```python
from build123d import *

# Parameters (mm, degrees)
SKETCH1_W           = 193
SKETCH1_H           = 10
BOSS_EXTRUDE1_DEPTH = 6
SKETCH4_W           = 16.888888889
SKETCH4_H           = 6
BOSS_EXTRUDE3_DEPTH = 6


with BuildPart() as part:
    # Sketch1 → Boss-Extrude1 (new body)
    with BuildSketch(Plane(origin=(0, 0, 0), x_dir=(1, 0, 0), z_dir=(0, 1, 0))):
        Rectangle(SKETCH1_W, SKETCH1_H)
    extrude(amount=BOSS_EXTRUDE1_DEPTH)

    # Sketch4 → Boss-Extrude3 (add)
    with BuildSketch(Plane.XZ):
        with Locations((-16.888888889, 8)):
            Rectangle(SKETCH4_W, SKETCH4_H)
        with Locations((-50.666666667, 8)):
            Rectangle(SKETCH4_W, SKETCH4_H)
    boss_extrude3 = extrude(amount=-BOSS_EXTRUDE3_DEPTH)

    # Mirror1: Boss-Extrude3 across plane
    add(boss_extrude3.mirror(Plane(origin=(0, 0, 0), x_dir=(0, 0, 1), z_dir=(1, 0, 0))))


solid = part.part
```
Input: part model. Units: mm. Frame: model coordinates. A direction names the side the tool comes from. Give positions to 0.01 mm unless a question says otherwise; leave off trailing zeros. Loops run counter-clockwise (first coordinate to the right, second up) from the corner with the lowest first, then second, coordinate; pieces in that order, holes last.
1) Section query B-B on y = 1.95. Return the cut outline in (x, z), and give its area (3 significant figures).
A:
outline: (-96.5, -5) - (96.5, -5) - (96.5, 5) - (59.11, 5) - (59.11, 11) - (42.22, 11) - (42.22, 5) - (25.33, 5) - (25.33, 11) - (8.44, 11) - (8.44, 5) - (-8.44, 5) - (-8.44, 11) - (-25.33, 11) - (-25.33, 5) - (-42.22, 5) - (-42.22, 11) - (-59.11, 11) - (-59.11, 5) - (-96.5, 5) - close
area: 2,340 mm2
2) Reachability of faces 1 (the flat face through (25.333, 3, 8)), 2 (the flat face through (-1, 0, 1)), 3 (the flat face through (59.111, 3, 8)) from +Z, -Z, +X, -X, +Y, -Y: full face, straight path, thin tool, end or side. Return the list, or none.
A:
face 1: +Z, +Y, -Y
face 2: +Z, -Z, +X, -X, -Y
face 3: +Z, +X, +Y, -Y
3) Contact query for flat-ended pins moving along their axis: pin 1 (3 mm diameter, centred on x = 73, y = 4.5, fed in from +Z); pin 2 (1.8 mm diameter, centred on y = 2.5, z = 8.5, fed in from -X); pin 3 (1.8 mm diameter, centred on y = 4.5, z = 8, fed in from +X); pin 4 (2 mm diameter, centred on x = 40, z = 7, fed in from -Y). Output: stop coordinate, or through.
A:
pin 1: stops at z = 5
pin 2: stops at x = -59.11
pin 3: stops at x = 59.11
pin 4: passes through
4) Mould query, pull axis X, two halves, no side actions, for faces 4 (the flat face through (8.444, 3, 8)), 5 (the flat face through (-59.111, 3, 8)), 6 (the flat face through (-78, 3, 5)). Classes: released by +X, released by -X, zero draft, split by the parting line, or undercut.
A:
face 4: undercut
face 5: released by -X
face 6: zero draft
5) Line query: L1, parallel to X at y = 3.9, z = 5.75; L2, parallel to Z at x = 84.5, y = 3.6. Output: solid intervals per line, ascending.
A:
L1: x = -59.11 to -42.22, -25.33 to -8.44, 8.44 to 25.33, 42.22 to 59.11
L2: z = -5 to 5
6) Section query C-C on x = 70. Return the cut outline in (y, z), and give its area (3 significant figures).
A:
outline: (0, -5) - (6, -5) - (6, 5) - (0, 5) - close
area: 60.0 mm2
7) Section query A-A on z = 7. Return the cut outline in (x, y).
A:
outline: (-59.11, 0) - (-42.22, 0) - (-42.22, 6) - (-59.11, 6) - close; (-25.33, 0) - (-8.44, 0) - (-8.44, 6) - (-25.33, 6) - close; (8.44, 0) - (25.33, 0) - (25.33, 6) - (8.44, 6) - close; (42.22, 0) - (59.11, 0) - (59.11, 6) - (42.22, 6) - close
